Build history of the part. All positions in model axes, mm. Face numbers are marked on the shaded views. A direction names the side the tool comes from. Give positions to 0.01 mm unless a question says otherwise; leave off trailing zeros. Order: outer loops, then holes, each group sorted by start corner. A loop starts at its lowest first (then second) coordinate and runs counter-clockwise, first axis right, second up. Notation, with made-up numbers: M -25.75,-11.5 L 28.25,-11.5 A23 ccw 28.25,2.5 Z; hole C 67,-4 d4. An arc over 180 degrees is marked long. Answer as CSV lines item,"result".
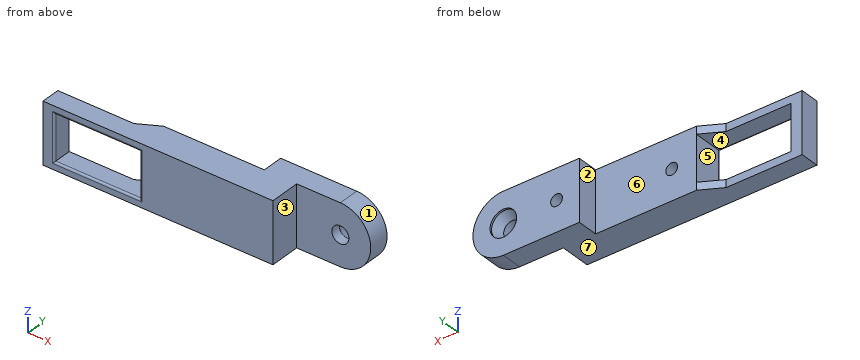
from build123d import *
from OCP.BRepFilletAPI import BRepFilletAPI_MakeChamfer

# Parameters (mm, degrees)
SKETCH1_W               = 34.25
SKETCH1_H               = 16
SKETCH1_W_2             = 22.5
SKETCH1_H_2             = 12
BOSS_EXTRUDE2_DEPTH     = 5
SKETCH4_W               = 16
SKETCH4_H               = 5
BOSS_EXTRUDE3_DEPTH     = 2
BOSS_EXTRUDE4_DEPTH     = 3
SKETCH6_R               = 1.55
CUT_EXTRUDE1_DEPTH      = 3.5
FILLET1_R               = 0.5
SKETCH8_W               = 25.75
SKETCH8_H               = 16
BOSS_EXTRUDE5_DEPTH     = 8
SKETCH9_W               = 10
SKETCH9_H               = 16
BOSS_EXTRUDE6_DEPTH     = 5.5
SKETCH10_R              = 1.55
CUT_EXTRUDE2_DEPTH      = 3.5
SKETCH11_W              = 16
SKETCH11_H              = 5.5
BOSS_EXTRUDE7_DEPTH     = 20
CUT_EXTRUDE3_DEPTH      = 70.543601431
CUT_EXTRUDE3_DEPTH_BACK = 70.543601431
SKETCH12_R              = 2.25
SKETCH13_R              = 3.5
CUT_EXTRUDE4_DEPTH      = 3
SKETCH14_W              = 1.5
SKETCH14_H              = 8
CUT_EXTRUDE5_DEPTH      = 70.002264456
CHAMFER1_SIZE2          = 1.25
CHAMFER1_SIZE           = 2.5
CHAMFER2_SIZE           = 5.5
CHAMFER2_SIZE_2         = 3


with BuildPart() as part:
    # Sketch1 → Boss-Extrude2 (new body)
    with BuildSketch(Plane(origin=(0, 0, 0), x_dir=(1, 0, 0), z_dir=(0, 1, 0))):
        with Locations((2.875, 0)):
            Rectangle(SKETCH1_W, SKETCH1_H)
        Rectangle(SKETCH1_W_2, SKETCH1_H_2, mode=Mode.SUBTRACT)
    extrude(amount=BOSS_EXTRUDE2_DEPTH)

    # Sketch4 → Boss-Extrude3 (add)
    with BuildSketch(Plane(origin=(20, 0, 0), x_dir=(0, 0, -1), z_dir=(1, 0, 0))):
        with Locations((0, 2.5)):
            Rectangle(SKETCH4_W, SKETCH4_H)
    extrude(amount=BOSS_EXTRUDE3_DEPTH)

    # Sketch3 → Boss-Extrude4 (add)
    with BuildSketch(Plane(origin=(0, 5, 0), x_dir=(1, 0, 0), z_dir=(0, 1, 0))):
        Polygon((5.75, 6), (11.25, 6), (11.25, -6), (5.75, -6), (5.75, -8), (22, -8), (22, 8), (5.75, 8), align=None)
    extrude(amount=BOSS_EXTRUDE4_DEPTH)

    # Sketch6 → Cut-Extrude1 (cut)
    with BuildSketch(Plane(origin=(0, 8, 0), x_dir=(1, 0, 0), z_dir=(0, 1, 0))):
        with Locations(Location((17.75, 0, 0), (0, 0, 270))):
            Circle(SKETCH6_R)
    extrude(amount=-CUT_EXTRUDE1_DEPTH, mode=Mode.SUBTRACT)

    # Fillet1
    fillet1_edges = [part.edges().sort_by_distance(p)[0] for p in [
        (11.25, 0, 0),
        (0, 0, -6),
        (-11.25, 0, 0),
        (0, 0, 6),
    ]]
    fillet(fillet1_edges, radius=FILLET1_R)

    # Sketch8 → Boss-Extrude5 (add)
    with BuildSketch(Plane(origin=(0, 8, 0), x_dir=(1, 0, 0), z_dir=(0, 1, 0))):
        with Locations((34.875, 0)):
            Rectangle(SKETCH8_W, SKETCH8_H)
    extrude(amount=-BOSS_EXTRUDE5_DEPTH)

    # Sketch9 → Boss-Extrude6 (add)
    with BuildSketch(Plane(origin=(0, 8, 0), x_dir=(1, 0, 0), z_dir=(0, 1, 0))):
        with Locations((42.75, 0)):
            Rectangle(SKETCH9_W, SKETCH9_H)
    extrude(amount=BOSS_EXTRUDE6_DEPTH)

    # Sketch10 → Cut-Extrude2 (cut)
    with BuildSketch(Plane(origin=(0, 13.5, 0), x_dir=(1, 0, 0), z_dir=(0, 1, 0))):
        with Locations(Location((43.75, 0, 0), (0, 0, 270))):
            Circle(SKETCH10_R)
    extrude(amount=-CUT_EXTRUDE2_DEPTH, mode=Mode.SUBTRACT)

    # Sketch11 → Boss-Extrude7 (add)
    with BuildSketch(Plane(origin=(47.75, 0, 0), x_dir=(0, 0, -1), z_dir=(1, 0, 0))):
        with Locations((0, 10.75)):
            Rectangle(SKETCH11_W, SKETCH11_H)
    extrude(amount=BOSS_EXTRUDE7_DEPTH)

    # Sketch12 → Cut-Extrude3 (cut, two sides: drawn at the far end of the back side and taken through both)
    with BuildSketch(Plane(origin=(0, 13.5, 0), x_dir=(1, 0, 0), z_dir=(0, 1, 0)).offset(-CUT_EXTRUDE3_DEPTH_BACK)):
        with Locations(Location((57.75, 0, 0), (0, 0, 270))):
            Circle(SKETCH12_R)
        with BuildLine():
            Line((57.75, 8), (67.75, 8))
            Line((67.75, 8), (67.75, -8))
            Line((67.75, -8), (57.75, -8))
            ThreePointArc((57.75, -8), (65.75, 0), (57.75, 8))
        make_face()
    extrude(amount=CUT_EXTRUDE3_DEPTH + CUT_EXTRUDE3_DEPTH_BACK, mode=Mode.SUBTRACT)

    # Sketch13 → Cut-Extrude4 (cut)
    with BuildSketch(Plane(origin=(0, 13.5, 0), x_dir=(1, 0, 0), z_dir=(0, 1, 0))):
        with Locations(Location((57.75, 0, 0), (0, 0, 270))):
            Circle(SKETCH13_R)
    extrude(amount=-CUT_EXTRUDE4_DEPTH, mode=Mode.SUBTRACT)

    # Sketch14 → Cut-Extrude5 (cut, through all)
    with BuildSketch(Plane(origin=(0, 0, -8), x_dir=(-1, 0, 0), z_dir=(0, 0, -1))):
        with Locations((-47, 4)):
            Rectangle(SKETCH14_W, SKETCH14_H)
    extrude(amount=-CUT_EXTRUDE5_DEPTH, mode=Mode.SUBTRACT)

    # Chamfer1
    chamfer1_edges = [part.edges().sort_by_distance(p)[0] for p in [
        (57.75, 10.5, -3.5),
    ]]
    chamfer1_side = [part.faces().sort_by_distance(p)[0] for p in [
        (57.75, 10.525, -3.5),
    ]]
    chamfer(chamfer1_edges, length=CHAMFER1_SIZE - 0.0001, length2=CHAMFER1_SIZE2 - 0.0001, reference=chamfer1_side[0])  # a hair under: the kernel refuses the full size

    # Chamfer2
    chamfer2_edges_1 = [part.edges().sort_by_distance(p)[0] for p in [
        (5.75, 8, 7),
    ]]
    chamfer2_side_1 = [part.faces().sort_by_distance(p)[0] for p in [
        (5.81, 8, 7),
    ]]
    chamfer2_edges_2 = [part.edges().sort_by_distance(p)[0] for p in [
        (5.75, 8, -7),
    ]]
    chamfer2_side_2 = [part.faces().sort_by_distance(p)[0] for p in [
        (5.81, 8, -7),
    ]]
    chamfer2 = BRepFilletAPI_MakeChamfer(part.part.solid().wrapped)
    for e in chamfer2_edges_1:
        chamfer2.Add(CHAMFER2_SIZE - 0.0001, CHAMFER2_SIZE_2 - 0.0001, e.wrapped, chamfer2_side_1[0].wrapped)
    for e in chamfer2_edges_2:
        chamfer2.Add(CHAMFER2_SIZE - 0.0001, CHAMFER2_SIZE_2 - 0.0001, e.wrapped, chamfer2_side_2[0].wrapped)
    add(Compound.cast(chamfer2.Shape()), mode=Mode.REPLACE)  # a hair under: the kernel refuses the full size


solid = part.part
Item 1: Band-saw the part on C-C (y = 2.5). Give the cut face in (x, z).
Geometry says:
outline,"M -14.25,-8 L 46.25,-8 L 46.25,8 L -14.25,8 Z; hole M -11.25,-6 L 11.25,-6 L 11.25,6 L -11.25,6 Z"
Item 2: Band-saw the part on D-D (x = 17.75). Give the cut face in (y, z).
Geometry says:
outline,"M 0,-8 L 8,-8 L 8,-1.55 L 4.5,-1.55 L 4.5,1.55 L 8,1.55 L 8,8 L 0,8 Z"
Item 3: 3-axis set-ups, long thin cutter, end or side, ignore diameter. For the marked faces 1, 2 and 3: which of +Z, -Z, +X, -X, +Y, -Y reach the whole face in a straight line?
Geometry says:
face 1,"+X, +Y, -Y"
face 2,"+Z, -Z, -X, +Y"
face 3,"+Z, -Z, +X, -Y"
Item 4: Drop flat-ended pins along their axis: pin 1 (3.5 mm diameter, centred on x = 17.75, z = 0, fed in from +Y); pin 2 (2.5 mm diameter, centred on y = 4, z = 4, fed in from +X); pin 3 (8 mm diameter, centred on x = -4.5, z = -2.5, fed in from +Y). Give the stop position or say it passes through.
Geometry says:
pin 1,"stops at y = 8"
pin 2,"stops at x = 46.25"
pin 3,"stops at y = 5"
Item 5: Band-saw the part on B-B (x = 0.5). Give the cut face in (y, z).
Geometry says:
outline,"M 0,-8 L 5,-8 L 5,-6 L 0.5,-6 A0.5 ccw 0,-6.5 Z; M 0,6.5 A0.5 ccw 0.5,6 L 5,6 L 5,8 L 0,8 Z"
Item 6: Pull direction Z, two halves, no side cores. Call the marked faces 4, 5, 6 and 7: released by +Z, released by -Z, zero draft, split by the parting line, or undercut.
Geometry says:
face 4,"undercut"
face 5,"undercut"
face 6,"zero draft"
face 7,"released by -Z"
Item 7: Probe line 1 along X through (y, z) = (13.3, 0); line 2 along X through (y, z) = (1.25, -4.25); line 3 along Z through (x, y) = (57.75, 9.1). List the from-to ranges inside material, lowest first. Write a range as from..to.
Geometry says:
line 1,"x = 37.75..42.2, 45.3..54.25, 61.25..65.75"
line 2,"x = -14.25..-11.25, 11.25..46.25"
line 3,"z = -8..-2.25, 2.25..8"
Item 8: Band-saw the part on A-A (z = 0). State how many separate pieces and enclosed holes the cut face has, and give its area (3 significant figures).
Geometry says:
separate pieces,"3"
enclosed holes,"0"
area,"398 mm2"
